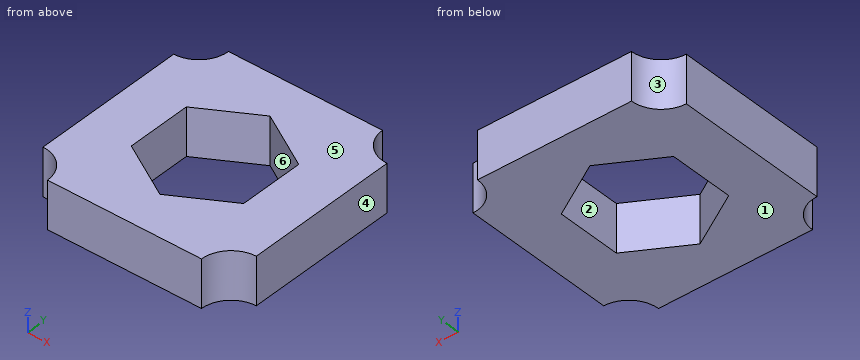
```python
from build123d import *

# Parameters (mm, degrees)
BOSS_EXTRUDE3_DEPTH = 10


with BuildPart() as part:
    # Sketch1 → Boss-Extrude3 (new, symmetric)
    with BuildSketch(Plane.XY):
        with BuildLine():
            Line((12.5, 0), (77.5, 0))
            ThreePointArc((77.5, 0), (81.161165235, 8.838834765), (90, 12.5))
            Line((90, 12.5), (90, 77.5))
            ThreePointArc((90, 77.5), (81.161165235, 81.161165235), (77.5, 90))
            Line((77.5, 90), (12.5, 90))
            ThreePointArc((12.5, 90), (8.838834765, 81.161165235), (0, 77.5))
            Line((0, 77.5), (0, 12.5))
            ThreePointArc((0, 12.5), (8.838834765, 8.838834765), (12.5, 0))
        make_face()
        Polygon((45, 72.378151261), (21.2898255, 58.68907563), (21.2898255, 31.31092437), (45, 17.621848739), (68.7101745, 31.31092437), (68.7101745, 58.68907563), align=None, mode=Mode.SUBTRACT)
    extrude(amount=BOSS_EXTRUDE3_DEPTH, both=True)


solid = part.part
```
The model under review builds one solid part; all positions refer to its coordinate system, in mm. Face numbers are marked on the shaded views. A direction names the side the tool comes from. Round coordinates to 2 decimals unless told otherwise and drop trailing zeros. Order: outer loops, then holes, each group sorted by start corner. A loop starts at its lowest first (then second) coordinate and runs counter-clockwise, first axis right, second up. Notation, with made-up numbers: (77.25, 2.5) -> (110.25, 2.5) arc R33 cw to (110.25, 30.5) -> close; hole circle Ø11 at (74, 38.5). An arc over 180 degrees is marked (long way). One line per item, written item: value. Start each with the question number.
Q1. Take a section at D-D (x = 7.5). Write out the cut boundary in (y, z), and give its area (3 significant figures).
Q2. Mouldability with a two-part tool opening along X and no side actions: class the marked faces 1, 2, 3 and 4 as released by +X, released by -X, zero draft, split by the parting line, or undercut.
Q3. Machinability: for the marked faces 5 and 6, which of the approach directions +Z, -Z, +X, -X, +Y, -Y give a long, thin tool a straight path to every point of the face, cutting with its end or side? Answer none if there is none.
Q4. Wall thickness on line 1 (X direction, y = 55, z = 4.75); line 2 (Y direction, x = 40, z = -7.5); line 3 (Y direction, x = 54.5, z = 0.75): over which ranges is each line inside the solid? List them lowest first.
Q5. Take a section at C-C (x = 28.5). Write out the cut boundary in (y, z), and give its area (3 significant figures).
Q6. Take a section at A-A (y = 46). Write out the cut boundary in (x, z), and give its area (3 significant figures).
Q7. Take a section at B-B (z = -6.25). Write out the cut boundary in (x, y).
Reported:
1. outline: (10, -10) -> (80, -10) -> (80, 10) -> (10, 10) -> close
1. area: 1,400 mm2
2. face 1: zero draft
2. face 2: undercut
2. face 3: released by -X
2. face 4: released by +X
3. face 5: +Z, +X, -X, +Y, -Y
3. face 6: +Z, -Z
4. line 1: x = 0 to 21.29, 68.71 to 90
4. line 2: y = 0 to 20.51, 69.49 to 90
4. line 3: y = 0 to 23.11, 66.89 to 90
5. outline: (0, -10) -> (27.15, -10) -> (27.15, 10) -> (0, 10) -> close; (62.85, -10) -> (90, -10) -> (90, 10) -> (62.85, 10) -> close
5. area: 1,090 mm2
6. outline: (0, -10) -> (21.29, -10) -> (21.29, 10) -> (0, 10) -> close; (68.71, -10) -> (90, -10) -> (90, 10) -> (68.71, 10) -> close
6. area: 852 mm2
7. outline: (0, 12.5) arc R12.5 cw to (12.5, 0) -> (77.5, 0) arc R12.5 cw to (90, 12.5) -> (90, 77.5) arc R12.5 cw to (77.5, 90) -> (12.5, 90) arc R12.5 cw to (0, 77.5) -> close; hole (21.29, 31.31) -> (45, 17.62) -> (68.71, 31.31) -> (68.71, 58.69) -> (45, 72.38) -> (21.29, 58.69) -> close
